```python
from build123d import *

# Parameters (mm, degrees)
SKETCH1_W           = 100
SKETCH1_H           = 20.5
SKETCH1_R           = 3.25
SKETCH1_R_2         = 1.5
BOSS_EXTRUDE1_DEPTH = 2
FILLET1_R           = 10.25


with BuildPart() as part:
    # Sketch1 → Boss-Extrude1 (new body)
    with BuildSketch(Plane(origin=(0, 0, 0), x_dir=(1, 0, 0), z_dir=(0, 1, 0))):
        with Locations((50, 10.25)):
            Rectangle(SKETCH1_W, SKETCH1_H)
        with Locations(Location((10.25, 10.25, 0), (0, 0, 270))):
            Circle(SKETCH1_R, mode=Mode.SUBTRACT)
        with Locations(Location((17.75, 10.25, 0), (0, 0, 270))):
            Circle(SKETCH1_R_2, mode=Mode.SUBTRACT)
        with Locations(Location((10.25, 17.75, 0), (0, 0, 90))):
            Circle(SKETCH1_R_2, mode=Mode.SUBTRACT)
        with Locations(Location((10.25, 2.75, 0), (0, 0, 90))):
            Circle(SKETCH1_R_2, mode=Mode.SUBTRACT)
        with Locations(Location((2.75, 10.25, 0), (0, 0, 270))):
            Circle(SKETCH1_R_2, mode=Mode.SUBTRACT)
        with Locations(Location((82.25, 10.25, 0), (0, 0, 90))):
            Circle(SKETCH1_R_2, mode=Mode.SUBTRACT)
        with Locations(Location((89.75, 17.75, 0), (0, 0, 270))):
            Circle(SKETCH1_R_2, mode=Mode.SUBTRACT)
        with Locations(Location((89.75, 2.75, 0), (0, 0, 270))):
            Circle(SKETCH1_R_2, mode=Mode.SUBTRACT)
        with Locations(Location((97.25, 10.25, 0), (0, 0, 90))):
            Circle(SKETCH1_R_2, mode=Mode.SUBTRACT)
        with Locations(Location((89.75, 10.25, 0), (0, 0, 90))):
            Circle(SKETCH1_R, mode=Mode.SUBTRACT)
    extrude(amount=BOSS_EXTRUDE1_DEPTH)

    # Fillet1
    fillet1_edges = [part.edges().sort_by_distance(p)[0] for p in [
        (0, 1, 0),
        (0, 1, -20.5),
        (100, 1, -20.5),
        (100, 1, 0),
    ]]
    fillet(fillet1_edges, radius=FILLET1_R - 0.0001)  # a hair under: the kernel refuses the full size


solid = part.part
```
Work out the finished part from the listing and answer in its coordinate system (mm). Round coordinates to 2 decimals unless told otherwise and drop trailing zeros. Write each loop counter-clockwise with the first axis right and the second up, starting at its lowest first coordinate (ties: lowest second). Pieces come first, ordered by that corner, then holes. Notation, with made-up numbers: (-17, 30) - (-8, 30) arc R9 cw to (-8, 46) - close; hole circle Ø4 at (11.25, -20). An arc over 180 degrees is marked (long way). Return JSON: item names as keys, results as strings. Group by question number.
Q1. The part is cut by section B-B on z = -3.25. Write down the section's boundary in (x, y), then the cut area to 3 significant figures.
Q2. The part is cut by section A-A on y = 0.75. Count the separate pieces of the cut face and the enclosed holes in it, then the cut area to 3 significant figures.
Q3. The mould has two halves that part along Z. Classify faces 1 (the cylindrical face through (91.237, 0.986, -2.945)), 2 (the cylindrical face through (2.923, 1.014, -3.082)), 3 (the cylindrical face through (10.18, 0.99, -16.25)), 4 (the flat face through (49, 1, -20.5)): released by +Z, released by -Z, zero draft, split by the parting line, or undercut.
Q4. The part is cut by section D-D on z = -17.75. Write down the section's boundary in (x, y).
Q5. Find the intervals of material crossed by L1, parallel to Z at x = 89.75, y = 1.45; L2, parallel to Z at x = 82.25, y = 1.15; L3, parallel to X at y = 0.75, z = -17.75, in increasing order.
Q6. The part is cut by section C-C on x = 2.75. Write down the section's boundary in (y, z).
Solved:
{
 "1": {"outline": "(2.76, 0) - (8.84, 0) - (8.84, 2) - (2.76, 2) - close; (11.66, 0) - (88.34, 0) - (88.34, 2) - (11.66, 2) - close; (91.16, 0) - (97.24, 0) - (97.24, 2) - (91.16, 2) - close", "area": "178 mm²"},
 "2": {"separate pieces": "1", "enclosed holes": "10", "area": "1,840 mm²"},
 "3": {"face 1": "undercut", "face 2": "released by +Z", "face 3": "undercut", "face 4": "released by -Z"},
 "4": {"outline": "(3.26, 0) - (8.75, 0) - (8.75, 2) - (3.26, 2) - close; (11.75, 0) - (88.25, 0) - (88.25, 2) - (11.75, 2) - close; (91.25, 0) - (96.74, 0) - (96.74, 2) - (91.25, 2) - close"},
 "5": {"L1": "-20.5 to -19.25, -16.25 to -13.5, -7 to -4.25, -1.25 to 0", "L2": "-20.5 to -11.75, -8.75 to 0", "L3": "3.26 to 8.75, 11.75 to 88.25, 91.25 to 96.74"},
 "6": {"outline": "(0, -17.24) - (2, -17.24) - (2, -11.75) - (0, -11.75) - close; (0, -8.75) - (2, -8.75) - (2, -3.26) - (0, -3.26) - close"}
}
